Autodesk Inventor part; units mm, degrees
ref_plane "Work Plane1" through (60.6806, 127.9398, 0) normal (1, 0, 0) x (0, 0, 1)
ref_plane "YZ Plane" through (0, 0, 0) normal (1, 0, 0) x (0, 1, 0)
ref_plane "XZ Plane" through (0, 0, 0) normal (0, 1, 0) x (-1, 0, 0)
sketch "Sketch1" plane through (0, 0, 0) normal (0, 0, 1) x (1, 0, 0)
  line L0 (29.0703, 0) -> (121.3612, 0)
  line L1 (121.3612, 0) -> (121.3612, 127.9398)
  line L2 (121.3612, 127.9398) -> (0, 127.9398)
  line L3 (0, 127.9398) -> (0, 13.0299)
  line L4 (0, 77.1398) -> (121.3612, 77.1398) construction
  line L5 (29.0703, 0) -> (29.0703, 26.0597) construction
  line L6 (92.2909, 0) -> (92.2909, 26.0597) construction
  line L7 (29.0703, 13.0299) -> (0, 13.0299) construction
  line L8 (92.2909, 13.0299) -> (121.3612, 13.0299) construction
  line L9 (0, 77.1398) -> (29.0703, 0)
  line L10 (92.2909, 0) -> (121.3612, 77.1398)
  point P0 (0, 0)
  dimension "d0" = 121.3612
  dimension "d1" = 127.9398
  dimension "d2" = 50.8
  dimension "d3" = 63.2206
extrude "Extrusion1" add sketch "Sketch1" along normal blind 6.35 contours L9 L3 L2 L1 L10 L0
sketch "Sketch2" plane through (0, 127.9398, 0) normal (0, 1, 0) x (1, 0, 0)
  line L0 (121.3612, 0) -> (0, 0) construction
  line L1 (0, 0) -> (0, -6.35) construction
  line L2 (121.3612, -6.35) -> (0, -6.35) construction
  line L3 (121.3612, 0) -> (121.3612, -6.35) construction
  line L4 (121.3612, -6.35) -> (0, -6.35) construction
  line L5 (60.6806, -6.35) -> (60.6806, 0) construction
  line L6 (121.3612, 0) -> (0, 0) construction
  circle A0 centre (60.6806, -3.175) radius 1.0541
  circle A1 centre (47.9806, -3.175) radius 1.0541
  circle A2 centre (35.2806, -3.175) radius 1.0541
  circle A3 centre (22.5806, -3.175) radius 1.0541
  circle A4 centre (9.8806, -3.175) radius 1.0541
  circle A5 centre (60.6806, -3.175) radius 1.0541
  circle A6 centre (73.3806, -3.175) radius 1.0541
  circle A7 centre (86.0806, -3.175) radius 1.0541
  circle A8 centre (98.7806, -3.175) radius 1.0541
  circle A9 centre (111.4806, -3.175) radius 1.0541
  dimension "d6" = 2.1082
  dimension "d9" = 12.7
extrude "Extrusion2" cut sketch "Sketch2" against normal blind 3.6322
sketch "Sketch3" plane through (121.3612, 77.1398, 0) normal (1, 0, 0) x (0, 0, -1)
  line L0 (0, 0) -> (0, 50.8) construction
  line L1 (0, 50.8) -> (-6.35, 50.8) construction
  line L2 (-6.35, 0) -> (-6.35, 50.8) construction
  line L3 (0, 0) -> (-6.35, 0) construction
  line L4 (0, 50.8) -> (-6.35, 50.8) construction
  line L5 (-3.175, 50.8) -> (-3.175, 0) construction
  line L6 (0, 0) -> (-6.35, 0) construction
  circle A0 centre (-3.175, 40.9194) radius 1.0541
  point P0 (0, -77.1398)
  dimension "d16" = 2.1082
  dimension "d17" = 9.8806
extrude "Extrusion3" cut sketch "Sketch3" against normal blind 25.4
pattern_linear "Rectangular Pattern1" count 3 spacing 12.7 along (0, -1, 0) of "Extrusion3"
ref_plane "Work Plane1" through (60.6806, 127.9398, 0) normal (1, 0, 0) x (0, 0, 1)
mirror "Mirror1" about plane through (60.6806, 127.9398, 0) normal (1, 0, 0) of "Extrusion3", "Rectangular Pattern1"
properties part number "top"
The listing builds one solid part. Answer for the finished solid, in the listing's coordinates (mm). Coordinates: 2 decimals unless noted, no trailing zeros. Write each loop counter-clockwise with the first axis right and the second up, starting at its lowest first coordinate (ties: lowest second). Pieces come first, ordered by that corner, then holes. Notation, with made-up numbers: (36.25, 40.5) - (40.25, 40.5) arc R29 ccw to (40.25, 71.5) - close; hole circle Ø2 at (63.25, 86.25). An arc over 180 degrees is marked (long way). One line per item, written item: value.
1) Find section D-D (y = 21.5). Give the vertices of the cut face in (x, z), and give its area (3 significant figures).
Geometry check:
outline: (20.97, 0) - (100.39, 0) - (100.39, 6.35) - (20.97, 6.35) - close
area: 504 mm2
2) Each of these flat-tipped pins is pushed along its axis until it touches: pin 1 Ø1.1 at (y, z) = (118, 2.5) entering from -X; pin 2 Ø1.7 at (y, z) = (118.06, 3.18) entering from -X; pin 3 Ø0.6 at (x, z) = (85.5, 3.5) entering from +Y. Where does it stop, or does it pass through?
Geometry check:
pin 1: stops at x = 0
pin 2: stops at x = 25.4
pin 3: stops at y = 124.31
3) Find section A-A (x = 106). Give the vertices of the cut face in (y, z) (3 decimals).
Geometry check:
outline: (36.378, 0) - (127.94, 0) - (127.94, 6.35) - (36.378, 6.35) - close; hole circle Ø2.108 at (92.659, 3.175); hole circle Ø2.108 at (105.359, 3.175); hole circle Ø2.108 at (118.059, 3.175)
4) Consider line 1 along X through (y, z) = (33, 2.25); line 2 along X through (y, z) = (41, 3.75). Determine where each line is inside the solid, lowest interval first. Write a range as from..to.
Geometry check:
line 1: x = 16.63..104.73
line 2: x = 13.62..107.74
5) Find section C-C (x = 17). Give the vertices of the cut face in (y, z) (3 decimals), and give its area (3 significant figures).
Geometry check:
outline: (32.029, 0) - (127.94, 0) - (127.94, 6.35) - (32.029, 6.35) - close; hole circle Ø2.108 at (92.659, 3.175); hole circle Ø2.108 at (105.359, 3.175); hole circle Ø2.108 at (118.059, 3.175)
area: 599 mm2
6) Find section B-B (y = 65.5). Give the vertices of the cut face in (x, z).
Geometry check:
outline: (4.39, 0) - (116.97, 0) - (116.97, 6.35) - (4.39, 6.35) - close
